Read the model definition and answer for the solid it produces. Units are mm, in the model's axes. Face numbers are marked on the shaded views. A direction names the side the tool comes from. Give positions to 0.01 mm unless a question says otherwise; leave off trailing zeros. Write each loop counter-clockwise with the first axis right and the second up, starting at its lowest first coordinate (ties: lowest second). Pieces come first, ordered by that corner, then holes. Notation, with made-up numbers: M -5,-33 L 11,-33 A10 cw 11,-18 Z; hole C 28,77.5 d2. An arc over 180 degrees is marked long. Use a Markdown table: item, result. Add a question column.
Item 1: Given P1, Ø3, axis at x = 18, z = -14, coming from the +Y side; P2, Ø1.5, axis at x = 53, y = 9.5, coming from the +Z side; P3, Ø4, axis at y = 3, z = 32.5, coming from the +X side; P4, Ø2.5, axis at y = 1.5, z = 5, coming from the -X side, each flat-ended and moving along its own axis, determine where each tip first touches the part or whether it passes through.
Item 2: A cutting plane is placed at A-A on x = 18. Determine the outline of the cut face in (y, z), then the cut area to 3 significant figures.
Item 3: Consider probe 1 along Z at (x, y) = (24, 2.75); probe 2 along Z at (x, y) = (-8, 7.75); probe 3 along Z at (x, y) = (-42, 1.6). Determine where each line is inside the solid, lowest interval first. Write a range as [from, to].
Item 4: The mould has two halves that part along X. Classify the marked faces 1, 2 and 3: pulls with the +X half, pulls with the -X half, needs draft (parallel to the pull), parting line crosses it, or undercut.
Item 5: A cutting plane is placed at D-D on y = 9.25. Count the separate pieces of the cut face and the enclosed holes in it, then the cut area to 3 significant figures.
Item 6: For the marked faces 4, 5, 6 and 7, determine the directions among +Z, -Z, +X, -X, +Y, -Y from which every point of the face is accessible in a straight line to the end or side of a thin tool.
Item 7: A cutting plane is placed at C-C on x = 60. Determine the outline of the cut face in (y, z), then the cut area to 3 significant figures.
Item 8: A cutting plane is placed at B-B on z = -3. Determine the outline of the cut face in (x, y), then the cut area to 3 significant figures.
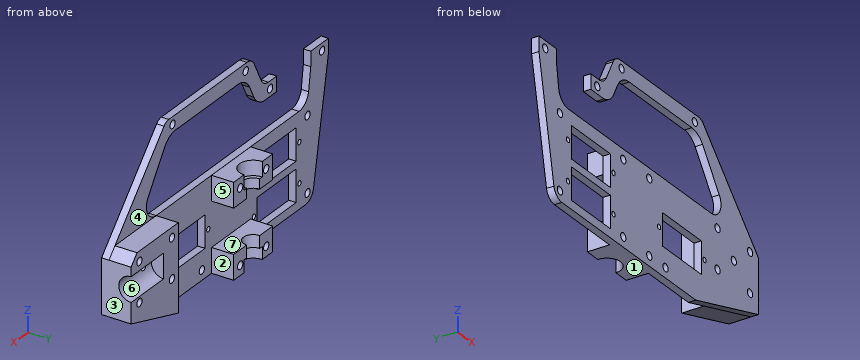
from build123d import *

# Parameters (mm, degrees)
SKETCH_1_R          = 1.6
SKETCH_1_R_2        = 1
SKETCH_1_W          = 24
SKETCH_1_H          = 13
EXTRUDE_1_DEPTH     = 3
SKETCH_2_R          = 1.6
SKETCH_2_W          = 24
SKETCH_2_H          = 10
EXTRUDE_2_DEPTH     = 9
SKETCH_3_R          = 5
CUT_EXTRUDE_1_DEPTH = 20
SKETCH_4_R          = 4
CUT_EXTRUDE_2_DEPTH = 72.704206567
SKETCH_6_R          = 5.6
CUT_EXTRUDE_3_DEPTH = 5
SKETCH_7_R          = 5.6
CUT_EXTRUDE_4_DEPTH = 6
FILLET_5_R          = 5
FILLET_6_R          = 5
SKETCH_8_W          = 21
SKETCH_8_H          = 6
CUT_EXTRUDE_5_DEPTH = 4.0000001


with BuildPart() as part:
    # Эскиз1 → Бобышка-Вытянуть1 (new body)
    with BuildSketch(Plane(origin=(0, 0, 0), x_dir=(1, 0, 0), z_dir=(0, 1, 0))):
        with BuildLine():
            Line((-59.846473334, -34), (-49.887758312, 18))
            Line((-49.887758312, 18), (36.612736258, 18))
            Line((36.612736258, 18), (75.112241688, 5.920216985))
            Line((75.112241688, 5.920216985), (75.112241688, -16.079783015))
            Line((75.112241688, -16.079783015), (41.245672077, -52.430849732))
            ThreePointArc((41.245672077, -52.430849732), (39.914841322, -53.372078747), (38.318998701, -53.704206567))
            Line((38.318998701, -53.704206567), (-9.799827382, -53.704206567))
            ThreePointArc((-9.799827382, -53.704206567), (-12.412320205, -52.967407389), (-14.254860003, -50.974159066))
            Line((-14.254860003, -50.974159066), (-19.846473334, -40))
            Line((-19.846473334, -40), (-59.846473334, -40))
            Line((-59.846473334, -40), (-59.846473334, -34))
        make_face()
        with Locations((-8, 14)):
            Circle(SKETCH_1_R, mode=Mode.SUBTRACT)
        with Locations((8, 14)):
            Circle(SKETCH_1_R, mode=Mode.SUBTRACT)
        with Locations((-8, -16)):
            Circle(SKETCH_1_R, mode=Mode.SUBTRACT)
        with Locations((8, -16)):
            Circle(SKETCH_1_R, mode=Mode.SUBTRACT)
        with Locations((-47, 14)):
            Circle(SKETCH_1_R, mode=Mode.SUBTRACT)
        with Locations((70, 0)):
            Circle(SKETCH_1_R, mode=Mode.SUBTRACT)
        with Locations((50, 0)):
            Circle(SKETCH_1_R, mode=Mode.SUBTRACT)
        with Locations((18, 14)):
            Circle(SKETCH_1_R, mode=Mode.SUBTRACT)
        with Locations((-47, -16)):
            Circle(SKETCH_1_R, mode=Mode.SUBTRACT)
        with Locations((-56, -37)):
            Circle(SKETCH_1_R, mode=Mode.SUBTRACT)
        with Locations((-24, -37)):
            Circle(SKETCH_1_R, mode=Mode.SUBTRACT)
        with Locations((50, -16)):
            Circle(SKETCH_1_R, mode=Mode.SUBTRACT)
        with Locations((70, -16)):
            Circle(SKETCH_1_R, mode=Mode.SUBTRACT)
        with Locations((-9, -50.704206567)):
            Circle(SKETCH_1_R, mode=Mode.SUBTRACT)
        with Locations((36, -50.704206567)):
            Circle(SKETCH_1_R, mode=Mode.SUBTRACT)
        with Locations((60, -8)):
            Circle(SKETCH_1_R, mode=Mode.SUBTRACT)
        with Locations((-42, -8)):
            Circle(SKETCH_1_R_2, mode=Mode.SUBTRACT)
        with Locations((-14, -8)):
            Circle(SKETCH_1_R_2, mode=Mode.SUBTRACT)
        with Locations((-42, 8)):
            Circle(SKETCH_1_R_2, mode=Mode.SUBTRACT)
        with Locations((-14, 8)):
            Circle(SKETCH_1_R_2, mode=Mode.SUBTRACT)
        with Locations((14, 0)):
            Circle(SKETCH_1_R_2, mode=Mode.SUBTRACT)
        with Locations((42, 0)):
            Circle(SKETCH_1_R_2, mode=Mode.SUBTRACT)
        with Locations((28, 0)):
            Rectangle(SKETCH_1_W, SKETCH_1_H, mode=Mode.SUBTRACT)
        with Locations((-28, 8)):
            Rectangle(SKETCH_1_W, SKETCH_1_H, mode=Mode.SUBTRACT)
        with Locations((-28, -8)):
            Rectangle(SKETCH_1_W, SKETCH_1_H, mode=Mode.SUBTRACT)
        with BuildLine():
            Line((-47.677053254, -24.900709984), (-49.000145857, -34))
            Line((-49.000145857, -34), (-22.297676486, -34))
            Line((-22.297676486, -34), (-19.846473334, -34))
            ThreePointArc((-19.846473334, -34), (-16.425778662, -35.467187694), (-13.988679802, -38.280431537))
            Line((-13.988679802, -38.280431537), (-11.413907263, -43.333707171))
            ThreePointArc((-11.413907263, -43.333707171), (-8.465843587, -46.522904488), (-4.28585507, -47.701783173))
            Line((-4.28585507, -47.701783173), (34.165827616, -47.701783173))
            ThreePointArc((34.165827616, -47.701783173), (37.877016972, -46.788889321), (40.741225842, -44.258551563))
            Line((40.741225842, -44.258551563), (51.02606102, -29.417576293))
            ThreePointArc((51.02606102, -29.417576293), (51.409841961, -23.216607983), (46.09451235, -20))
            Line((46.09451235, -20), (-41.778616049, -20))
            ThreePointArc((-41.778616049, -20), (-45.612951708, -21.385038456), (-47.677053254, -24.900709984))
        make_face(mode=Mode.SUBTRACT)
    extrude(amount=EXTRUDE_1_DEPTH)

    # Эскиз2 → Бобышка-Вытянуть2 (add)
    with BuildSketch(Plane(origin=(0, 3, 0), x_dir=(1, 0, 0), z_dir=(0, 1, 0))):
        Polygon((46.101706289, 15.022696844), (46.09451235, -20), (71.459960933, -20), (75.112241688, -16.079783015), (75.112241688, 5.920216985), align=None)
        with Locations((50, 0)):
            Circle(SKETCH_2_R, mode=Mode.SUBTRACT)
        with Locations((70, 0)):
            Circle(SKETCH_2_R, mode=Mode.SUBTRACT)
        with Locations((70, -16)):
            Circle(SKETCH_2_R, mode=Mode.SUBTRACT)
        with Locations((50, -16)):
            Circle(SKETCH_2_R, mode=Mode.SUBTRACT)
        with Locations((60, -8)):
            Circle(SKETCH_2_R, mode=Mode.SUBTRACT)
        with Locations((0, 13)):
            Rectangle(SKETCH_2_W, SKETCH_2_H)
        with Locations((-8, 14)):
            Circle(SKETCH_2_R, mode=Mode.SUBTRACT)
        with Locations((8, 14)):
            Circle(SKETCH_2_R, mode=Mode.SUBTRACT)
        with Locations((0, -14.961092538)):
            Rectangle(SKETCH_2_W, SKETCH_2_H)
        with Locations((-8, -16)):
            Circle(SKETCH_2_R, mode=Mode.SUBTRACT)
        with Locations((8, -16)):
            Circle(SKETCH_2_R, mode=Mode.SUBTRACT)
    extrude(amount=EXTRUDE_2_DEPTH)

    # Эскиз3 → Вырез-Вытянуть1 (cut)
    with BuildSketch(Plane(origin=(75.112241688, 0, 0), x_dir=(0, 0, -1), z_dir=(1, 0, 0))):
        with Locations((-7.384625177, 12)):
            Circle(SKETCH_3_R)
    extrude(amount=-CUT_EXTRUDE_1_DEPTH, mode=Mode.SUBTRACT)

    # Эскиз4 → Вырез-Вытянуть2 (cut, through all)
    with BuildSketch(Plane(origin=(0, 0, -18), x_dir=(-1, 0, 0), z_dir=(0, 0, -1))):
        with Locations((0, 12)):
            Circle(SKETCH_4_R)
    extrude(amount=-CUT_EXTRUDE_2_DEPTH, mode=Mode.SUBTRACT)

    # Эскиз6 → Вырез-Вытянуть3 (cut)
    with BuildSketch(Plane(origin=(0, 0, -18), x_dir=(-1, 0, 0), z_dir=(0, 0, -1))):
        with Locations((0, 12)):
            Circle(SKETCH_6_R)
    extrude(amount=-CUT_EXTRUDE_3_DEPTH, mode=Mode.SUBTRACT)

    # Эскиз7 → Вырез-Вытянуть4 (cut)
    with BuildSketch(Plane.XY.offset(19.961092538)):
        with Locations((0, 12)):
            Circle(SKETCH_7_R)
    extrude(amount=-CUT_EXTRUDE_4_DEPTH, mode=Mode.SUBTRACT)

    # Скругление5
    fillet_5_edges = [part.edges().sort_by_distance(p)[0] for p in [
        (-49.887758312, 1.5, -18),
    ]]
    fillet(fillet_5_edges, radius=FILLET_5_R)

    # Скругление6
    fillet_6_edges = [part.edges().sort_by_distance(p)[0] for p in [
        (-19.846473334, 1.5, 40),
    ]]
    fillet(fillet_6_edges, radius=FILLET_6_R)

    # Эскиз8 → Вырез-Вытянуть5 (cut, through all)
    with BuildSketch(Plane(origin=(0, 3, 0), x_dir=(1, 0, 0), z_dir=(0, 1, 0))):
        with Locations((-38.500145857, -37)):
            Rectangle(SKETCH_8_W, SKETCH_8_H)
    extrude(amount=-CUT_EXTRUDE_5_DEPTH, mode=Mode.SUBTRACT)


solid = part.part
Filled in:
| question | item | result |
|---|---|---|
| 1 | P1 | through |
| 1 | P2 | z = 20 |
| 1 | P3 | x = 61.68 |
| 1 | P4 | x = -54.53 |
| 2 | outline | M 0,-18 L 3,-18 L 3,-15.6 L 0,-15.6 Z; M 0,-12.4 L 3,-12.4 L 3,-6.5 L 0,-6.5 Z; M 0,6.5 L 3,6.5 L 3,20 L 0,20 Z; M 0,47.7 L 3,47.7 L 3,53.7 L 0,53.7 Z |
| 2 | area | 83.4 mm² |
| 3 | probe 1 | [-18, -6.5], [6.5, 20], [47.7, 53.7] |
| 3 | probe 2 | [-18, -15.6], [-12.4, -8], [9.96, 14.4], [17.6, 19.96] |
| 3 | probe 3 | [-18, -9], [-7, 7], [9, 20] |
| 4 | face 1 | needs draft |
| 4 | face 2 | undercut |
| 4 | face 3 | pulls with the +X half |
| 5 | separate pieces | 5 |
| 5 | enclosed holes | 8 |
| 5 | area | 966 mm² |
| 6 | face 4 | +Z, +X, -X, +Y |
| 6 | face 5 | +Z, -Z, +Y |
| 6 | face 6 | +X, +Y |
| 6 | face 7 | -X, +Y |
| 7 | outline | M 0,-10.66 L 12,-10.66 L 12,2.38 A5 cw 7.1,6.4 L 0,6.4 Z; M 0,9.6 L 7.52,9.6 A5 cw 12,12.38 L 12,20 L 3,20 L 3,32.3 L 0,32.3 Z |
| 7 | area | 343 mm² |
| 8 | outline | M -52.76,0 L -40,0 L -40,3 L -52.76,3 Z; M -16,0 L 16,0 L 16,3 L -16,3 Z; M 40,0 L 75.11,0 L 75.11,12 L 46.1,12 L 46.1,3 L 40,3 Z |
| 8 | area | 501 mm² |
